from build123d import *

# Parameters (mm, degrees)
SKETCH1_W           = 100
SKETCH1_H           = 35
BOSS_EXTRUDE1_DEPTH = 50
SKETCH4_R           = 12.5
CUT_EXTRUDE2_DEPTH  = 100
SKETCH5_W           = 15
SKETCH5_H           = 5
SKETCH5_W_2         = 10
CUT_EXTRUDE3_DEPTH  = 25


with BuildPart() as part:
    # Sketch1 → Boss-Extrude1 (new body)
    with BuildSketch(Plane.XY):
        with Locations((50, 17.5)):
            Rectangle(SKETCH1_W, SKETCH1_H)
    extrude(amount=BOSS_EXTRUDE1_DEPTH)

    # Sketch4 → Cut-Extrude2 (cut)
    with BuildSketch(Plane(origin=(100, 0, 0), x_dir=(0, 0, -1), z_dir=(1, 0, 0))):
        with Locations((-25, 35)):
            Circle(SKETCH4_R)
    extrude(amount=-CUT_EXTRUDE2_DEPTH, mode=Mode.SUBTRACT)

    # Sketch5 → Cut-Extrude3 (cut)
    with BuildSketch(Plane.XY.offset(50)):
        with Locations((7.5, 32.5)):
            Rectangle(SKETCH5_W, SKETCH5_H)
        with Locations((30, 32.5)):
            Rectangle(SKETCH5_W_2, SKETCH5_H)
        with Locations((70, 32.5)):
            Rectangle(SKETCH5_W_2, SKETCH5_H)
        with Locations((92.5, 32.5)):
            Rectangle(SKETCH5_W, SKETCH5_H)
        with Locations((50, 32.5)):
            Rectangle(SKETCH5_W_2, SKETCH5_H)
    extrude(amount=-CUT_EXTRUDE3_DEPTH, mode=Mode.SUBTRACT)


solid = part.part
The listing builds one solid part. Answer for the finished solid, in the listing's coordinates (mm). A direction names the side the tool comes from. Round coordinates to 2 decimals unless told otherwise and drop trailing zeros. Write each loop counter-clockwise with the first axis right and the second up, starting at its lowest first coordinate (ties: lowest second). Pieces come first, ordered by that corner, then holes. Notation, with made-up numbers: M -4.5,46.25 L 27.5,46.25 A21 cw 27.5,82.25 Z; hole C 27.25,15.25 d7. An arc over 180 degrees is marked long. Write each question's results on one line, items separated by ' | '. Start each with the question number.
(1) For faces 4 (the flat face through (65, 32, 43)), 5 (the flat face through (92, 30, 43)), 6 (the flat face through (49, 0, 25)), 7 (the flat face through (15, 32, 43)), 8 (the flat face through (0, 13, 25)), determine the directions among +Z, -Z, +X, -X, +Y, -Y from which every point of the face is accessible in a straight line to the end or side of a thin tool.
(2) The part is cut by section D-D, the plane x = 68. Write down the section's boundary in (y, z).
(3) The part is cut by section B-B, the plane x = 36. Write down the section's boundary in (y, z).
(4) The part is cut by section A-A, the plane y = 33. Write down the section's boundary in (x, z).
(5) Determine the mould class of faces 1 (the flat face through (75, 32, 43)), 2 (the flat face through (49, 35, 6)), 3 (the flat face through (100, 13, 25)) for opening direction X: +X half, -X half, draft (parallel to the pull), parting line (faces both ways), or undercut.
(6) Each of these flat-tipped pins is pushed along its axis until it touches: P1, Ø5, axis at x = 68, z = 45, coming from the +Y side; P2, Ø1.5, axis at y = 32, z = 45.5, coming from the +X side; P3, Ø4, axis at y = 33.5, z = 42.5, coming from the -X side. Where does it stop, or does it pass through?
(7) The part is cut by section C-C, the plane z = 39. Write down the section's boundary in (x, y), and give its area (3 significant figures).
(8) Find the intervals of material crossed by line 1 (X direction, y = 33, z = 45.5); line 2 (Y direction, x = 92, z = 38.5); line 3 (Z direction, x = 21, y = 26), in increasing order.
Worked answers:
1) face 4: +Z, +Y | face 5: +Z, +X, +Y | face 6: +Z, -Z, +X, -X, -Y | face 7: +Z, -X, +Y | face 8: +Z, -Z, -X, +Y, -Y
2) outline: M 0,0 L 35,0 L 35,12.5 A12.5 cw 30,36.46 L 30,50 L 0,50 Z
3) outline: M 0,0 L 35,0 L 35,12.5 A12.5 cw 35,37.5 L 35,50 L 0,50 Z
4) outline: M 0,0 L 100,0 L 100,12.66 L 0,12.66 Z; M 15,37.34 L 25,37.34 L 25,50 L 15,50 Z; M 35,37.34 L 45,37.34 L 45,50 L 35,50 Z; M 55,37.34 L 65,37.34 L 65,50 L 55,50 Z; M 75,37.34 L 85,37.34 L 85,50 L 75,50 Z
5) face 1: undercut | face 2: draft | face 3: +X half
6) P1: stops at y = 30 | P2: stops at x = 85 | P3: stops at x = 15
7) outline: M 0,0 L 100,0 L 100,30 L 85,30 L 85,35 L 75,35 L 75,30 L 65,30 L 65,35 L 55,35 L 55,30 L 45,30 L 45,35 L 35,35 L 35,30 L 25,30 L 25,35 L 15,35 L 15,30 L 0,30 Z | area: 3,200 mm²
8) line 1: x = 15 to 25, 35 to 45, 55 to 65, 75 to 85 | line 2: y = 0 to 30 | line 3: z = 0 to 16.33, 33.67 to 50
